Check sheet for the drawn part. Datum: minimum x, y, z corner. Units: mm. A direction names the side the tool comes from. Round coordinates to 2 decimals unless told otherwise and drop trailing zeros. Write each loop counter-clockwise with the first axis right and the second up, starting at its lowest first coordinate (ties: lowest second). Pieces come first, ordered by that corner, then holes. Notation, with made-up numbers: M 3.5,22.5 L 42.5,22.5 A30 cw 42.5,46.5 Z; hole C -30.5,70.25 d5. An arc over 180 degrees is marked long. Put each result on its own line as item: value.
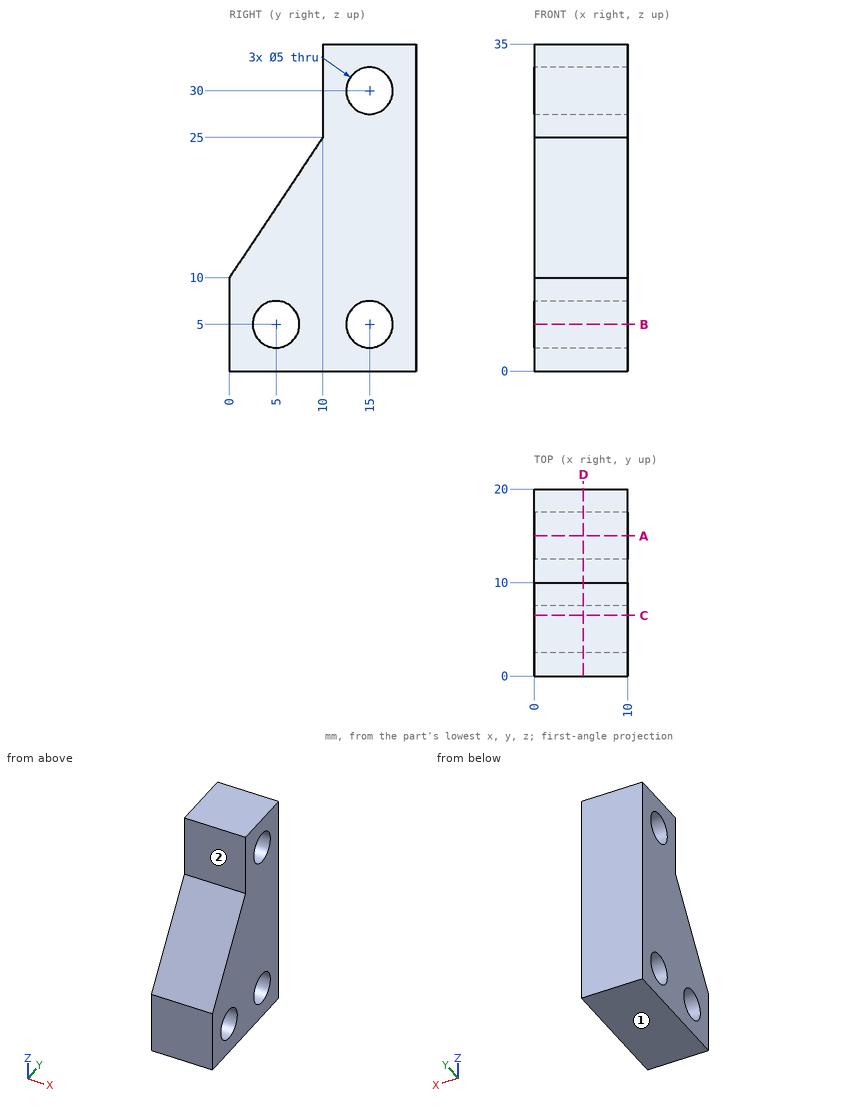
1. Access from +Z, -Z, +X, -X, +Y, -Y to the whole of each face (thin tool, end or side, straight path). Record for the marked faces 1 and 2.
Computed values:
face 1: -Z, +X, -X, +Y, -Y
face 2: +Z, +X, -X, -Y
2. Cross-section at A-A (y = 15). Enter the section's corners in (x, z).
Computed values:
outline: M 0,0 L 10,0 L 10,2.5 L 0,2.5 Z; M 0,7.5 L 10,7.5 L 10,27.5 L 0,27.5 Z; M 0,32.5 L 10,32.5 L 10,35 L 0,35 Z
3. Cross-section at C-C (y = 6.5). Enter the section's corners in (x, z).
Computed values:
outline: M 0,0 L 10,0 L 10,3 L 0,3 Z; M 0,7 L 10,7 L 10,19.75 L 0,19.75 Z
4. Scan lines: probe 1 along Y at (x, z) = (4.25, 5); probe 2 along Y at (x, z) = (7.25, 30); probe 3 along Y at (x, z) = (2.25, 28.5). Record each from-to range of solid material in increasing order.
Computed values:
probe 1: y = 0 to 2.5, 7.5 to 12.5, 17.5 to 20
probe 2: y = 10 to 12.5, 17.5 to 20
probe 3: y = 10 to 13, 17 to 20
5. Cross-section at B-B (z = 5). Enter the section's corners in (x, y), then the cut area to 3 significant figures.
Computed values:
outline: M 0,0 L 10,0 L 10,2.5 L 0,2.5 Z; M 0,7.5 L 10,7.5 L 10,12.5 L 0,12.5 Z; M 0,17.5 L 10,17.5 L 10,20 L 0,20 Z
area: 100 mm2
6. Depth check by flat-ended pin: pin 1 Ø3 at (y, z) = (15, 5) entering from +X; pin 2 Ø5 at (x, z) = (1, 16) entering from -Y. Enter the tip coordinate at first touch or a pass-through.
Computed values:
pin 1: passes through
pin 2: stops at y = 2.33
7. Cross-section at D-D (x = 5.25). Enter the section's corners in (y, z), then the cut area to 3 significant figures.
Computed values:
outline: M 0,0 L 20,0 L 20,35 L 10,35 L 10,25 L 0,10 Z; hole C 5,5 d5; hole C 15,5 d5; hole C 15,30 d5
area: 466 mm2
